```python
from build123d import *

# Parameters (mm, degrees)
SKETCH1_R           = 14.2875
BOSS_EXTRUDE1_DEPTH = 3.175
FILLET1_R           = 20
FILLET2_R           = 20


with BuildPart() as part:
    # Sketch1 → Boss-Extrude1 (new body)
    with BuildSketch(Plane.XY):
        with BuildLine():
            Line((-205.8238, 0), (-165.0238, -40.8))
            ThreePointArc((-165.0238, -40.8), (-136.173843328, 28.849956672), (-205.8238, 0))
        make_face()
        with Locations((-165.0238, 0)):
            Circle(SKETCH1_R, mode=Mode.SUBTRACT)
        with BuildLine():
            ThreePointArc((-205.8238, 0), (-136.173843328, 28.849956672), (-165.0238, -40.8))
            Line((-165.0238, -40.8), (-134.758308099, -40.8))
            ThreePointArc((-134.758308099, -40.8), (-119.646895144, -22.838049517), (-114.2238, 0))
            ThreePointArc((-114.2238, 0), (-149.086422549, 48.235256815), (-205.8238, 30.265491901))
            Line((-205.8238, 30.265491901), (-205.8238, 0))
        make_face()
        with BuildLine():
            ThreePointArc((-114.2238, 0), (-119.646895144, -22.838049517), (-134.758308099, -40.8))
            Line((-134.758308099, -40.8), (-30.265491901, -40.8))
            ThreePointArc((-30.265491901, -40.8), (-22.838049517, 45.376904856), (50.8, 0))
            ThreePointArc((50.8, 0), (45.376904856, -22.838049517), (30.265491901, -40.8))
            Line((30.265491901, -40.8), (134.758308099, -40.8))
            ThreePointArc((134.758308099, -40.8), (129.102775516, 35.921024484), (205.8238, 30.265491901))
            Line((205.8238, 30.265491901), (205.8238, 52))
            Line((205.8238, 52), (-205.8238, 52))
            Line((-205.8238, 52), (-205.8238, 30.265491901))
            ThreePointArc((-205.8238, 30.265491901), (-149.086422549, 48.235256815), (-114.2238, 0))
        make_face()
        with BuildLine():
            ThreePointArc((50.8, 0), (-22.838049517, 45.376904856), (-30.265491901, -40.8))
            Line((-30.265491901, -40.8), (30.265491901, -40.8))
            ThreePointArc((30.265491901, -40.8), (45.376904856, -22.838049517), (50.8, 0))
        make_face()
        Circle(SKETCH1_R, mode=Mode.SUBTRACT)
        with BuildLine():
            Line((205.8238, 0), (165.0238, -40.8))
            ThreePointArc((165.0238, -40.8), (136.173843328, 28.849956672), (205.8238, 0))
        make_face()
        with Locations((165.0238, 0)):
            Circle(SKETCH1_R, mode=Mode.SUBTRACT)
        with BuildLine():
            ThreePointArc((205.8238, 30.265491901), (129.102775516, 35.921024484), (134.758308099, -40.8))
            Line((134.758308099, -40.8), (165.0238, -40.8))
            ThreePointArc((165.0238, -40.8), (136.173843328, 28.849956672), (205.8238, 0))
            Line((205.8238, 0), (205.8238, 30.265491901))
        make_face()
    extrude(amount=BOSS_EXTRUDE1_DEPTH)

    # Fillet1
    fillet1_edges = [part.edges().sort_by_distance(p)[0] for p in [
        (-205.8238, 52, 1.5875),
        (205.8238, 52, 1.5875),
    ]]
    fillet(fillet1_edges, radius=FILLET1_R)

    # Fillet2
    fillet2_edges = [part.edges().sort_by_distance(p)[0] for p in [
        (-205.8238, 0, 1.5875),
        (205.8238, 0, 1.5875),
        (165.0238, -40.8, 1.5875),
        (-165.0238, -40.8, 1.5875),
    ]]
    fillet(fillet2_edges, radius=FILLET2_R)


solid = part.part
```
Here's how the part is built. I have some questions about the finished solid (model axes, mm). Coordinates: 2 decimals unless noted, no trailing zeros. Loops run counter-clockwise (first coordinate to the right, second up) from the corner with the lowest first, then second, coordinate; pieces in that order, holes last. Notation, with made-up numbers: (67.5, 51) -> (124.5, 51) arc R21 ccw to (124.5, 67) -> close; hole circle Ø9 at (31.25, 36.25). An arc over 180 degrees is marked (long way). Return JSON: item names as keys, results as strings.
1) If we section it at C-C, the plane y = 0: Write out the boundary of the cut face in (x, z) (1 decimal), then the cut area to 3 significant figures.
Results below:
{"outline": "(-204, 0) -> (-179.3, 0) -> (-179.3, 3.2) -> (-204, 3.2) -> close; (-150.7, 0) -> (-14.3, 0) -> (-14.3, 3.2) -> (-150.7, 3.2) -> close; (14.3, 0) -> (150.7, 0) -> (150.7, 3.2) -> (14.3, 3.2) -> close; (179.3, 0) -> (204, 0) -> (204, 3.2) -> (179.3, 3.2) -> close", "area": "1,020 mm²"}
2) Will this pin go through, and if not, where does the flat tip stop? pin 1 (23 mm diameter, centred on x = 165.02, y = 0, fed in from +Z).
Results below:
{"pin 1": "through"}
3) If we section it at B-B, the plane z = 2.35: Write out the boundary of the cut face in (x, y) (1 decimal).
Results below:
{"outline": "(-205.8, 8.3) arc R20 ccw to (-200, -5.9) -> (-170.9, -34.9) arc R20 ccw to (-156.7, -40.8) -> (156.7, -40.8) arc R20 ccw to (170.9, -34.9) -> (200, -5.9) arc R20 ccw to (205.8, 8.3) -> (205.8, 32) arc R20 ccw to (185.8, 52) -> (-185.8, 52) arc R20 ccw to (-205.8, 32) -> close; hole circle Ø28.6 at (-165, 0); hole circle Ø28.6 at (0, 0); hole circle Ø28.6 at (165, 0)"}
4) I need wall thicknesses on line 1 (Y direction, x = -0.5, z = 1.9); line 2 (Y direction, x = -12.5, z = 2.2); line 3 (Y direction, x = 188, z = 1.6). Which ranges of each line are inside material? Lowest first, please. Write a range as from..to.
Results below:
{"line 1": "-40.8..-14.28, 14.28..52", "line 2": "-40.8..-6.92, 6.92..52", "line 3": "-17.82..51.88"}
5) Thinking about a two-plate mould opening in X: for faces 1 (the face through (-3, 17, 0)), 2 (the face through (-179.3, 0.6, 1.6)), 3 (the face through (-185.627, -20.196, 1.565)), 4 (the face through (178.222, -5.472, 1.565)), which applies, +X half, -X half, draft (parallel to the pull), parting line (faces both ways), or undercut?
Results below:
{"face 1": "draft", "face 2": "undercut", "face 3": "-X half", "face 4": "undercut"}
6) If we section it at A-A, the plane x = 0: Write out the boundary of the cut face in (y, z) (1 decimal).
Results below:
{"outline": "(-40.8, 0) -> (-14.3, 0) -> (-14.3, 3.2) -> (-40.8, 3.2) -> close; (14.3, 0) -> (52, 0) -> (52, 3.2) -> (14.3, 3.2) -> close"}
